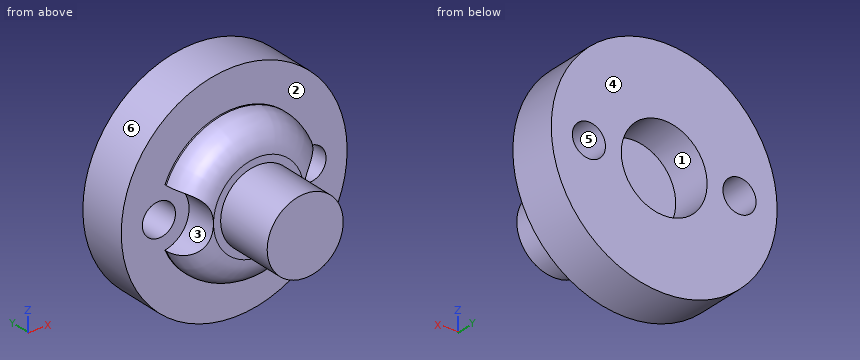
Autodesk Inventor part; units mm, degrees
ref_plane "YZ Plane" through (0, 0, 0) normal (1, 0, 0) x (0, 1, 0)
ref_plane "XZ Plane" through (0, 0, 0) normal (0, 1, 0) x (-1, 0, 0)
ref_plane "XY Plane" through (0, 0, 0) normal (0, 0, 1) x (1, 0, 0)
sketch "Sketch1" plane through (0, 0, 0) normal (0, 1, 0) x (-1, 0, 0)
  circle A0 centre (0, 0) radius 2.525
  dimension "d0" = 5.05
extrude "Extrusion1" add sketch "Sketch1" along normal blind 4
sketch "Sketch2" plane through (0, 4, 0) normal (0, 1, 0) x (1, 0, 0)
  circle A0 centre (0, 0) radius 5
  dimension "d3" = 10
extrude "Extrusion2" add sketch "Sketch2" along normal blind 5.4
fillet "Fillet1" radius 2 1 edges at (-5, 4, 0)
sketch "Sketch3" plane through (0, 9.4, 0) normal (0, 1, 0) x (1, 0, 0)
  circle A0 centre (0, 0) radius 7.5
  circle A1 centre (0, 0) radius 6.25
  circle A2 centre (0, 0) radius 5
  circle A3 centre (-5, 0) radius 1.1
  circle A4 centre (5, 0) radius 1.1
  point P0 (4.879, -1.0933)
  point P1 (-4.879, -1.0933)
  point P2 (-4.879, 1.0933)
  point P3 (4.879, 1.0933)
  dimension "d7" = 15
  dimension "d8" = 12.5
  dimension "d9" = 2.2
  dimension "d10" = 2.2
extrude "Extrusion3" add sketch "Sketch3" against normal blind 3.3 contours A0 | A1
extrude "Extrusion4" cut sketch "Sketch3" against normal blind 5.4 contours A2 A4 | A2 A4 | A3 A2 | A2 A3
sketch "Sketch4" plane through (0, 6.1, 0) normal (0, -1, 0) x (1, 0, 0)
  arc A0 (4.879, -1.0933) -> (4.879, 1.0933) centre (5, 0) ccw
  arc A1 (-4.879, 1.0933) -> (-4.879, -1.0933) centre (-5, 0) ccw
  circle A2 centre (-5, 0) radius 2
  circle A3 centre (0, 0) radius 3
  circle A4 centre (5, 0) radius 2
extrude "Extrusion5" cut sketch "Sketch4" along normal blind 3.3 contours A2 | A4
sketch "Sketch5" plane through (0, 0, 0) normal (1, 0, 0) x (0, 1, 0)
  point P0 (0, 0)
sketch "Sketch6" plane through (0, 9.4, 0) normal (0, 1, 0) x (1, 0, 0)
  circle A0 centre (0, 0) radius 2.85
  dimension "d17" = 5.7
extrude "Extrusion6" cut sketch "Sketch6" against normal blind 2.7
properties part number "spinner_under_3DPrint"
Geometry: final body of the model. Coordinates: model frame, mm. Face numbers are marked on the shaded views. A direction names the side the tool comes from. Round coordinates to 2 decimals unless told otherwise and drop trailing zeros. Loops run counter-clockwise (first coordinate to the right, second up) from the corner with the lowest first, then second, coordinate; pieces in that order, holes last.
Q1. Section A-A on x = -5. Return loops of the section in (y, z).
Q2. Section B-B on x = 0. Return loops of the section in (y, z) (3 decimals), plus the area to 3 significant figures.
Q3. Material intervals for L1, parallel to X at y = 7.95, z = 0; L2, parallel to Z at x = 0, y = 7.75; L3, parallel to Y at x = -4.25, z = -3.25, sorted ascending.
Q4. Section C-C on y = 0.5. Return loops of the section in (x, z) (3 decimals).
Q5. Pull-direction query (Z, two-part tool) for the marked faces 4, 5 and 6; classes: released by +Z, released by -Z, zero draft, split by the parting line, or undercut.
Q6. Section D-D on z = 0.5. State how many separate pieces and enclosed holes the cut face has, plus the area to 3 significant figures.
Q7. Pin query (flat end, axial travel): P1, Ø5, axis at y = 8, z = 4, coming from the -X side; P2, Ø4.5, axis at x = 0, z = 0, coming from the +Y side; P3, Ø1, axis at x = 4, z = -2.5, coming from the -Y side; P4, Ø1.8, axis at x = 5, z = 0, coming from the -Y side. Return the tip coordinate at first contact, or that it passes through.
Q8. Access query for the marked faces 1, 2 and 3. Directions: +Z, -Z, +X, -X, +Y, -Y. A direction counts if a zero-diameter tool reaches every point of the face in a straight line with its end or side. Return the directions, or none.
Evaluation:
1. outline: (6.1, -5.59) - (9.4, -5.59) - (9.4, -1.1) - (6.1, -1.1) - close; (6.1, 1.1) - (9.4, 1.1) - (9.4, 5.59) - (6.1, 5.59) - close
2. outline: (0, -2.525) - (4, -2.525) - (4, -3) arc R2 ccw to (6, -5) - (6.1, -5) - (6.1, -7.5) - (9.4, -7.5) - (9.4, -2.85) - (6.7, -2.85) - (6.7, 2.85) - (9.4, 2.85) - (9.4, 7.5) - (6.1, 7.5) - (6.1, 5) - (6, 5) arc R2 ccw to (4, 3) - (4, 2.525) - (0, 2.525) - close
2. area: 73.6 mm2
3. L1: x = -7.5 to -6.1, -3.9 to -2.85, 2.85 to 3.9, 6.1 to 7.5
3. L2: z = -7.5 to -2.85, 2.85 to 7.5
3. L3: y = 6.1 to 9.4
4. outline: circle Ø5.05 at (0, 0)
5. face 4: zero draft
5. face 5: undercut
5. face 6: split by the parting line
6. separate pieces: 3
6. enclosed holes: 0
6. area: 54.0 mm2
7. P1: stops at x = -7.35
7. P2: stops at y = 6.7
7. P3: stops at y = 4.41
7. P4: passes through
8. face 1: +Y
8. face 2: -Y
8. face 3: -X, -Y
